Verification items for the finished model (mm, model axes). A direction names the side the tool comes from. Coordinates: 2 decimals unless noted, no trailing zeros. Order: outer loops, then holes, each group sorted by start corner. A loop starts at its lowest first (then second) coordinate and runs counter-clockwise, first axis right, second up.
Q1. Depth check by flat-ended pin: P1, Ø2, axis at x = 6, z = 19, coming from the +Y side; P2, Ø6, axis at y = -34, z = 132.5, coming from the +X side; P3, Ø6, axis at x = 31.5, y = -21, coming from the +Z side. Enter the tip coordinate at first touch or a pass-through.
Q2. Cross-section at A-A, the plane y = 4.5. Record the boundary of the cut face in (x, z), and give its area (3 significant figures).
Q3. Cross-section at C-C, the plane x = -19. Record the boundary of the cut face in (y, z).
Q4. Draft check along Z on faces 1 (the cylindrical face through (-0.932, 27.954, 1.749)), 2 (the flat face through (-1, -8, 152.4)), 3 (the flat face through (-38.442, 5, 23)), 4 (the flat face through (0, -21.002, 23)). Enter one of: pulls with the +Z half, pulls with the -Z half, needs draft (parallel to the pull), parting line crosses it, or undercut.
Q5. Thickness scan on line 1 (Z direction, x = -3, y = -19.5); line 2 (Z direction, x = 37, y = -14); line 3 (X direction, y = 18.5, z = 70). Record the ranges inside material, lowest first.
Q6. Set-up check for faces 5 (the flat face through (-38.69, 5, 129)), 6 (the cylindrical face through (-49.642, 27.954, 75.502)): record each of +Z, -Z, +X, -X, +Y, -Y from which the full face is reachable in a straight line by a thin tool's end or side.
Q7. Cross-section at B-B, the plane z = 98. Record the boundary of the cut face in (x, y).
Q8. Cross-section at D-D, the plane y = -28. Record the boundary of the cut face in (x, z).
from build123d import *

# Parameters (mm, degrees)
F0_W         = 101.6
F0_H         = 76.2
F1_DEPTH     = 152.4
F2_W         = 76.2
F2_H         = 25.4
F3_DEPTH     = 50.8
F4_R         = 26.3680405282
F5_T1_DEPTH  = 48.8639189435
F5_T3_DEPTH  = 99.6639189435
F5_T6_ANGLE  = 90
F5_T8_ANGLE  = 90
F5_T10_ANGLE = 90
F5_T12_ANGLE = 90
F5_T14_ANGLE = 90
F5_T16_ANGLE = 90
F5_T18_ANGLE = 90
F5_T20_ANGLE = 90


# Not quite as in the source:
# - a fillet or chamfer that OpenCascade refuses, or shapes differently, is made with other operations: its cross-section is extruded or revolved along the edge and cut away or added


with BuildPart() as f1:
    # F0 (on Top) → F1 (new body)
    with BuildSketch(Plane.XY):
        with Locations((-0.5902759731, -8.3016921655)):
            Rectangle(F0_W, F0_H)
    extrude(amount=F1_DEPTH)

    # F2 (on face) → F3 (cut)
    with BuildSketch(Plane(origin=(0, 29.7983078345, 0), x_dir=(-1, 0, 0), z_dir=(0, 1, 0))):
        with Locations((0.5902759731, 129.54)):
            Rectangle(F2_W, F2_H)
        with Locations((0.5074083115, 93.9800965559)):
            Rectangle(F2_W, F2_H)
        with Locations((0.42454065, 58.4201931119)):
            Rectangle(F2_W, F2_H)
        with Locations((0.3416729884, 22.8602896678)):
            Rectangle(F2_W, F2_H)
    extrude(amount=-F3_DEPTH, mode=Mode.SUBTRACT)

    # F4
    f4_edges = [f1.edges().sort_by_distance(p)[0] for p in [
        (-51.390276, -8.301692, 152.4),
        (50.209724, -8.301692, 152.4),
        (-51.390276, -8.301692, 0),
        (50.209724, -8.301692, 0),
    ]]
    fillet(f4_edges, radius=F4_R)

    # F5: fillet of radius 6.1321024484 on 16 edges, made by hand

    # F5_s2 → F5_t1 (cut)
    with BuildSketch(Plane.YZ.offset(-25.0222354448)):
        with BuildLine():
            ThreePointArc((23.6662053861, 152.4), (28.0022566103, 150.6039487758), (29.7983078345, 146.2678975516))
            Line((29.7983078345, 146.2678975516), (29.7983078345, 152.4))
            Line((29.7983078345, 152.4), (23.6662053861, 152.4))
        make_face()
        with BuildLine():
            ThreePointArc((-46.4016921655, 146.2678975516), (-44.6056409413, 150.6039487758), (-40.2695897171, 152.4))
            Line((-40.2695897171, 152.4), (-46.4016921655, 152.4))
            Line((-46.4016921655, 152.4), (-46.4016921655, 146.2678975516))
        make_face()
        with BuildLine():
            ThreePointArc((23.6662053861, 0), (28.0022566103, 1.7960512242), (29.7983078345, 6.1321024484))
            Line((29.7983078345, 6.1321024484), (29.7983078345, 0))
            Line((29.7983078345, 0), (23.6662053861, 0))
        make_face()
        with BuildLine():
            ThreePointArc((-46.4016921655, 6.1321024484), (-44.6056409413, 1.7960512242), (-40.2695897171, 0))
            Line((-40.2695897171, 0), (-46.4016921655, 0))
            Line((-46.4016921655, 0), (-46.4016921655, 6.1321024484))
        make_face()
    extrude(amount=F5_T1_DEPTH, mode=Mode.SUBTRACT)

    # F5_s4 → F5_t3 (cut)
    with BuildSketch(Plane.XY.offset(26.3680405282)):
        with BuildLine():
            ThreePointArc((-45.2581735247, -46.4016921655), (-49.5942247489, -44.6056409413), (-51.3902759731, -40.2695897171))
            Line((-51.3902759731, -40.2695897171), (-51.3902759731, -46.4016921655))
            Line((-51.3902759731, -46.4016921655), (-45.2581735247, -46.4016921655))
        make_face()
        with BuildLine():
            ThreePointArc((44.0776215785, -46.4016921655), (48.4136728027, -44.6056409413), (50.2097240269, -40.2695897171))
            Line((50.2097240269, -40.2695897171), (50.2097240269, -46.4016921655))
            Line((50.2097240269, -46.4016921655), (44.0776215785, -46.4016921655))
        make_face()
        with BuildLine():
            ThreePointArc((-51.3902759731, 23.6662053861), (-49.5942247489, 28.0022566103), (-45.2581735247, 29.7983078345))
            Line((-45.2581735247, 29.7983078345), (-51.3902759731, 29.7983078345))
            Line((-51.3902759731, 29.7983078345), (-51.3902759731, 23.6662053861))
        make_face()
        with BuildLine():
            ThreePointArc((50.2097240269, 23.6662053861), (48.4136728027, 28.0022566103), (44.0776215785, 29.7983078345))
            Line((44.0776215785, 29.7983078345), (50.2097240269, 29.7983078345))
            Line((50.2097240269, 29.7983078345), (50.2097240269, 23.6662053861))
        make_face()
    extrude(amount=F5_T3_DEPTH, mode=Mode.SUBTRACT)

    # F5_s5 → F5_t6 (revolve, cut)
    with BuildSketch(Plane.XY.offset(26.3680405282)):
        with BuildLine():
            ThreePointArc((-45.2581735247, -46.4016921655), (-49.5942247489, -44.6056409413), (-51.3902759731, -40.2695897171))
            Line((-51.3902759731, -40.2695897171), (-51.3902759731, -46.4016921655))
            Line((-51.3902759731, -46.4016921655), (-45.2581735247, -46.4016921655))
        make_face()
    revolve(axis=Axis((-25.0222354448, -46.4016921655, 26.3680405282), (0, -1, 0)), revolution_arc=F5_T6_ANGLE, mode=Mode.SUBTRACT)

    # F5_s7 → F5_t8 (revolve, cut)
    with BuildSketch(Plane.XY.offset(126.0319594718)):
        with BuildLine():
            ThreePointArc((-45.2581735247, -46.4016921655), (-49.5942247489, -44.6056409413), (-51.3902759731, -40.2695897171))
            Line((-51.3902759731, -40.2695897171), (-51.3902759731, -46.4016921655))
            Line((-51.3902759731, -46.4016921655), (-45.2581735247, -46.4016921655))
        make_face()
    revolve(axis=Axis((-25.0222354448, -46.4016921655, 126.0319594718), (0, 1, 0)), revolution_arc=F5_T8_ANGLE, mode=Mode.SUBTRACT)

    # F5_s9 → F5_t10 (revolve, cut)
    with BuildSketch(Plane.XY.offset(26.3680405282)):
        with BuildLine():
            ThreePointArc((44.0776215785, -46.4016921655), (48.4136728027, -44.6056409413), (50.2097240269, -40.2695897171))
            Line((50.2097240269, -40.2695897171), (50.2097240269, -46.4016921655))
            Line((50.2097240269, -46.4016921655), (44.0776215785, -46.4016921655))
        make_face()
    revolve(axis=Axis((23.8416834987, -46.4016921655, 26.3680405282), (0, 1, 0)), revolution_arc=F5_T10_ANGLE, mode=Mode.SUBTRACT)

    # F5_s11 → F5_t12 (revolve, cut)
    with BuildSketch(Plane.XY.offset(126.0319594718)):
        with BuildLine():
            ThreePointArc((44.0776215785, -46.4016921655), (48.4136728027, -44.6056409413), (50.2097240269, -40.2695897171))
            Line((50.2097240269, -40.2695897171), (50.2097240269, -46.4016921655))
            Line((50.2097240269, -46.4016921655), (44.0776215785, -46.4016921655))
        make_face()
    revolve(axis=Axis((23.8416834987, -46.4016921655, 126.0319594718), (0, -1, 0)), revolution_arc=F5_T12_ANGLE, mode=Mode.SUBTRACT)

    # F5_s13 → F5_t14 (revolve, cut)
    with BuildSketch(Plane.XY.offset(26.3680405282)):
        with BuildLine():
            ThreePointArc((-51.3902759731, 23.6662053861), (-49.5942247489, 28.0022566103), (-45.2581735247, 29.7983078345))
            Line((-45.2581735247, 29.7983078345), (-51.3902759731, 29.7983078345))
            Line((-51.3902759731, 29.7983078345), (-51.3902759731, 23.6662053861))
        make_face()
    revolve(axis=Axis((-25.0222354448, 29.7983078345, 26.3680405282), (0, -1, 0)), revolution_arc=F5_T14_ANGLE, mode=Mode.SUBTRACT)

    # F5_s15 → F5_t16 (revolve, cut)
    with BuildSketch(Plane.XY.offset(126.0319594718)):
        with BuildLine():
            ThreePointArc((-51.3902759731, 23.6662053861), (-49.5942247489, 28.0022566103), (-45.2581735247, 29.7983078345))
            Line((-45.2581735247, 29.7983078345), (-51.3902759731, 29.7983078345))
            Line((-51.3902759731, 29.7983078345), (-51.3902759731, 23.6662053861))
        make_face()
    revolve(axis=Axis((-25.0222354448, 29.7983078345, 126.0319594718), (0, 1, 0)), revolution_arc=F5_T16_ANGLE, mode=Mode.SUBTRACT)

    # F5_s17 → F5_t18 (revolve, cut)
    with BuildSketch(Plane.XY.offset(26.3680405282)):
        with BuildLine():
            ThreePointArc((50.2097240269, 23.6662053861), (48.4136728027, 28.0022566103), (44.0776215785, 29.7983078345))
            Line((44.0776215785, 29.7983078345), (50.2097240269, 29.7983078345))
            Line((50.2097240269, 29.7983078345), (50.2097240269, 23.6662053861))
        make_face()
    revolve(axis=Axis((23.8416834987, 29.7983078345, 26.3680405282), (0, 1, 0)), revolution_arc=F5_T18_ANGLE, mode=Mode.SUBTRACT)

    # F5_s19 → F5_t20 (revolve, cut)
    with BuildSketch(Plane.XY.offset(126.0319594718)):
        with BuildLine():
            ThreePointArc((50.2097240269, 23.6662053861), (48.4136728027, 28.0022566103), (44.0776215785, 29.7983078345))
            Line((44.0776215785, 29.7983078345), (50.2097240269, 29.7983078345))
            Line((50.2097240269, 29.7983078345), (50.2097240269, 23.6662053861))
        make_face()
    revolve(axis=Axis((23.8416834987, 29.7983078345, 126.0319594718), (0, -1, 0)), revolution_arc=F5_T20_ANGLE, mode=Mode.SUBTRACT)


solid = f1.part
Check values:
1. P1: stops at y = -21
1. P2: stops at x = 49.98
1. P3: stops at z = 151.99
2. outline: (-51.39, 26.37) arc R26.37 ccw to (-25.02, 0) - (23.84, 0) arc R26.37 ccw to (50.21, 26.37) - (50.21, 126.03) arc R26.37 ccw to (23.84, 152.4) - (-25.02, 152.4) arc R26.37 ccw to (-51.39, 126.03) - close; hole (-38.69, 116.84) - (37.51, 116.84) - (37.51, 142.24) - (-38.69, 142.24) - close; hole (-38.61, 81.28) - (37.59, 81.28) - (37.59, 106.68) - (-38.61, 106.68) - close; hole (-38.52, 45.72) - (37.68, 45.72) - (37.68, 71.12) - (-38.52, 71.12) - close; hole (-38.44, 10.16) - (37.76, 10.16) - (37.76, 35.56) - (-38.44, 35.56) - close
2. area: 7,150 mm2
3. outline: (-46.4, 6.13) arc R6.13 ccw to (-40.27, 0) - (23.67, 0) arc R6.13 ccw to (29.8, 6.13) - (29.8, 10.16) - (-21, 10.16) - (-21, 35.56) - (29.8, 35.56) - (29.8, 45.72) - (-21, 45.72) - (-21, 71.12) - (29.8, 71.12) - (29.8, 81.28) - (-21, 81.28) - (-21, 106.68) - (29.8, 106.68) - (29.8, 116.84) - (-21, 116.84) - (-21, 142.24) - (29.8, 142.24) - (29.8, 146.27) arc R6.13 ccw to (23.67, 152.4) - (-40.27, 152.4) arc R6.13 ccw to (-46.4, 146.27) - close
4. face 1: pulls with the -Z half
4. face 2: pulls with the +Z half
4. face 3: undercut
4. face 4: undercut
5. line 1: z = 0 to 10.16, 35.56 to 45.72, 71.12 to 81.28, 106.68 to 116.84, 142.24 to 152.4
5. line 2: z = 3.52 to 10.16, 35.56 to 45.72, 71.12 to 81.28, 106.68 to 116.84, 142.24 to 148.88
5. line 3: x = -51.39 to -38.52, 37.68 to 50.21
6. face 5: +Y
6. face 6: +Z, -Z, -X, +Y
7. outline: (-51.39, -40.27) arc R6.13 ccw to (-45.26, -46.4) - (44.08, -46.4) arc R6.13 ccw to (50.21, -40.27) - (50.21, 23.67) arc R6.13 ccw to (44.08, 29.8) - (37.59, 29.8) - (37.59, -21) - (-38.61, -21) - (-38.61, 29.8) - (-45.26, 29.8) arc R6.13 ccw to (-51.39, 23.67) - close
8. outline: (-51.39, 26.37) arc R26.37 ccw to (-25.02, 0) - (23.84, 0) arc R26.37 ccw to (50.21, 26.37) - (50.21, 126.03) arc R26.37 ccw to (23.84, 152.4) - (-25.02, 152.4) arc R26.37 ccw to (-51.39, 126.03) - close
